Drawing for the job (mm, zero at the part's lowest x, y, z). A direction names the side the tool comes from. Round coordinates to 2 decimals unless told otherwise and drop trailing zeros. Loops run counter-clockwise (first coordinate to the right, second up) from the corner with the lowest first, then second, coordinate; pieces in that order, holes last. Notation, with made-up numbers: M -29,84 L -12,84 A17 ccw -12,93 Z; hole C 39,61 d9. An arc over 180 degrees is marked long. Answer in a Markdown table with one row per item.
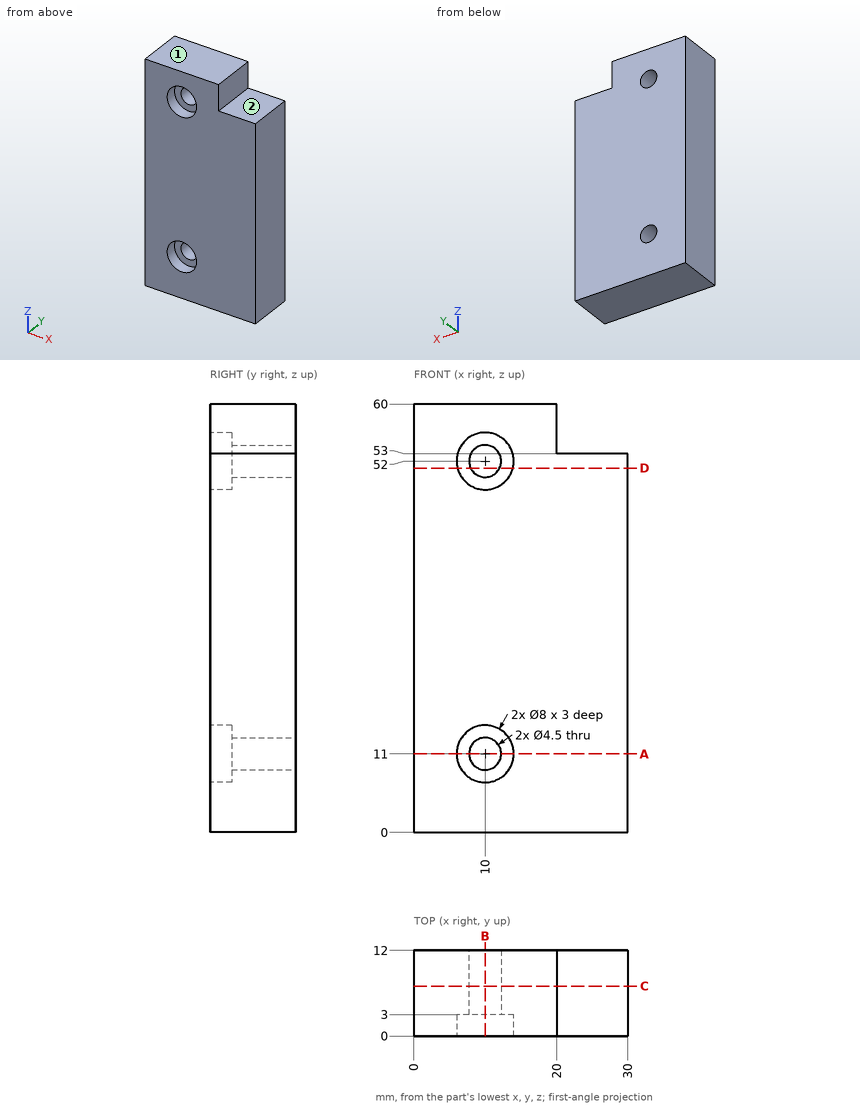
1. Wall check: probe 1 along Z at (x, y) = (10, 2.3); probe 2 along Z at (x, y) = (10, 5.25); probe 3 along Z at (x, y) = (24.5, 7). Give the ranges that are in metal, low to high.
Verdict:
| item | result |
|---|---|
| probe 1 | z = 0 to 7, 15 to 48, 56 to 60 |
| probe 2 | z = 0 to 8.75, 13.25 to 49.75, 54.25 to 60 |
| probe 3 | z = 0 to 53 |
2. Saw through at D-D (z = 51). Write the cut outline in (x, y), and give its area (3 significant figures).
Verdict:
| item | result |
|---|---|
| outline | M 0,0 L 6.13,0 L 6.13,3 L 7.98,3 L 7.98,12 L 0,12 Z; M 12.02,3 L 13.87,3 L 13.87,0 L 30,0 L 30,12 L 12.02,12 Z |
| area | 300 mm² |
3. Tool access for the marked faces 1 and 2: list every direction of +Z, -Z, +X, -X, +Y, -Y with a clear straight run to the whole face (end or side of a thin tool).
Verdict:
| item | result |
|---|---|
| face 1 | +Z, +X, -X, +Y, -Y |
| face 2 | +Z, +X, +Y, -Y |
4. Saw through at A-A (z = 11). Write the cut outline in (x, y), and give its area (4 significant figures).
Verdict:
| item | result |
|---|---|
| outline | M 0,0 L 6,0 L 6,3 L 7.75,3 L 7.75,12 L 0,12 Z; M 12.25,3 L 14,3 L 14,0 L 30,0 L 30,12 L 12.25,12 Z |
| area | 295.5 mm² |
5. Saw through at B-B (x = 10). Write the cut outline in (y, z).
Verdict:
| item | result |
|---|---|
| outline | M 0,0 L 12,0 L 12,8.75 L 3,8.75 L 3,7 L 0,7 Z; M 0,15 L 3,15 L 3,13.25 L 12,13.25 L 12,49.75 L 3,49.75 L 3,48 L 0,48 Z; M 0,56 L 3,56 L 3,54.25 L 12,54.25 L 12,60 L 0,60 Z |
6. Pin check, flat tips, straight feed: pin 1 (2.5 mm diameter, centred on x = 9.5, z = 13, fed in from -Y); pin 2 (3 mm diameter, centred on x = 26.5, y = 6, fed in from +Z). Stop position of each tip, or through.
Verdict:
| item | result |
|---|---|
| pin 1 | stops at y = 3 |
| pin 2 | stops at z = 53 |
7. Saw through at C-C (y = 7). Write the cut outline in (x, z), and give its area (3 significant figures).
Verdict:
| item | result |
|---|---|
| outline | M 0,0 L 30,0 L 30,53 L 20,53 L 20,60 L 0,60 Z; hole C 10,11 d4.5; hole C 10,52 d4.5 |
| area | 1,700 mm² |
